from build123d import *

# Parameters (mm, degrees)
F0_W     = 37.592
F0_H     = 16.637
F1_DEPTH = 2.286
F2_W     = 16.002
F2_H     = 8.4582
F3_DEPTH = 2.413
F4_W     = 2.6162
F4_H     = 5.334
F5_DEPTH = 17.1196
F6_R     = 0.508


with BuildPart() as f1:
    # F0 (on Top) → F1 (new body)
    with BuildSketch(Plane.XY):
        with Locations((18.796, 8.3185)):
            Rectangle(F0_W, F0_H)
    extrude(amount=F1_DEPTH)

    # F2 (on face) → F3 (join)
    with BuildSketch(Plane.XY.offset(2.286)):
        with Locations((18.542, 6.6421)):
            Rectangle(F2_W, F2_H)
    extrude(amount=F3_DEPTH)

    # F4 (on face) → F5 (join)
    with BuildSketch(Plane(origin=(0, 0, 0), x_dir=(1, 0, 0), z_dir=(0, 0, -1))):
        with Locations((1.5621, -11.2776)):
            Rectangle(F4_W, F4_H)
    extrude(amount=F5_DEPTH)

    # F6
    f6_edges = [f1.edges().sort_by_distance(p)[0] for p in [
        (2.8702, 13.9446, -8.5598),
        (0.254, 13.9446, -8.5598),
        (2.8702, 8.6106, -8.5598),
        (0.254, 8.6106, -8.5598),
    ]]
    fillet(f6_edges, radius=F6_R)


solid = f1.part
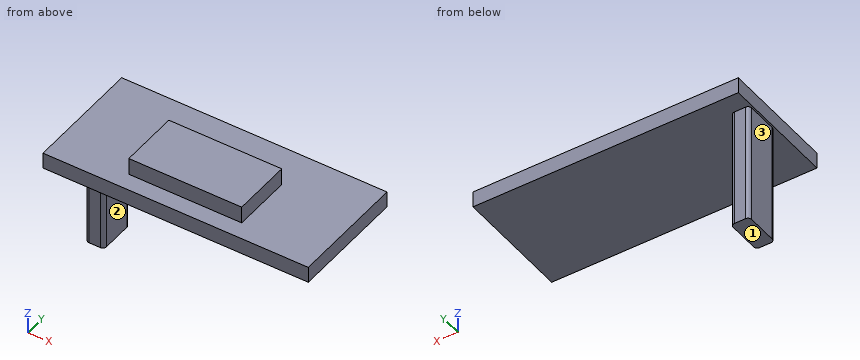
Work out the finished part from the listing and answer in its coordinate system (mm). Face numbers are marked on the shaded views. A direction names the side the tool comes from. Round coordinates to 2 decimals unless told otherwise and drop trailing zeros. Order: outer loops, then holes, each group sorted by start corner. A loop starts at its lowest first (then second) coordinate and runs counter-clockwise, first axis right, second up. Notation, with made-up numbers: M 49.25,-35 L 70.25,-35 A20 ccw 70.25,-4 Z; hole C 39,43.5 d9. An arc over 180 degrees is marked long. One line per item, written item: value.
Q1. Flat-ended cylindrical pins translate along their axes: pin 1 (0.7 mm diameter, centred on x = 16, z = 3.5, fed in from -Y); pin 2 (0.8 mm diameter, centred on x = 2, z = -10.5, fed in from -Y); pin 3 (0.7 mm diameter, centred on y = 7.5, z = 3.5, fed in from +X); pin 4 (1.5 mm diameter, centred on y = 6.5, z = -10, fed in from -X). Find the tip coordinate at first contact, or state that the pin passes through.
Derived:
pin 1: y = 2.41
pin 2: y = 8.61
pin 3: x = 26.54
pin 4: through
Q2. For the marked faces 1, 2 and 3, determine the directions among +Z, -Z, +X, -X, +Y, -Y from which every point of the face is accessible in a straight line to the end or side of a thin tool.
Derived:
face 1: -Z, +X, -X, +Y, -Y
face 2: -Z, +X, +Y, -Y
face 3: -Z, -X, +Y, -Y
Q3. Find section C-C on x = 28. Write down the section's boundary in (y, z), then the cut area to 3 significant figures.
Derived:
outline: M 0,0 L 16.64,0 L 16.64,2.29 L 0,2.29 Z
area: 38.0 mm²
Q4. Find section A-A on y = 3.5. Write down the section's boundary in (x, z).
Derived:
outline: M 0,0 L 37.59,0 L 37.59,2.29 L 26.54,2.29 L 26.54,4.7 L 10.54,4.7 L 10.54,2.29 L 0,2.29 Z
Q5. Find section B-B on x = 24. Write down the section's boundary in (y, z), then the cut area to 3 significant figures.
Derived:
outline: M 0,0 L 16.64,0 L 16.64,2.29 L 10.87,2.29 L 10.87,4.7 L 2.41,4.7 L 2.41,2.29 L 0,2.29 Z
area: 58.4 mm²
Q6. Straight lines are drawn through the part: line 1 (X direction, y = 7.75, z = 3); line 2 (Z direction, x = 18.5, y = 15); line 3 (X direction, y = 13.5, z = -15.25). For each, find the intervals that lie inside material, in ascending order.
Derived:
line 1: 10.54 to 26.54
line 2: 0 to 2.29
line 3: 0.26 to 2.87
